Design review of the part built by this model. Coordinates are the model's own, in mm. A direction names the side the tool comes from. Round coordinates to 2 decimals unless told otherwise and drop trailing zeros. Loops run counter-clockwise (first coordinate to the right, second up) from the corner with the lowest first, then second, coordinate; pieces in that order, holes last. Notation, with made-up numbers: (-32, 84.25) - (-27, 84.25) arc R7 cw to (-27, 90.25) - close; hole circle Ø6 at (75.5, 44). An arc over 180 degrees is marked (long way). Return JSON: item names as keys, results as strings. Group by question number.
(1) We need section B-B, the plane y = 13.2. Write out the cut boundary in (x, z).
(2) For faces 5 (the flat face through (27, 25, 1.5)), 6 (the cylindrical face through (-0.2, 13.1, 9.6)), 7 (the flat face through (1, 3, 2.2)), 8 (the flat face through (21, 22.4, -1)), list the 3-axis set-ups (+Z, -Z, +X, -X, +Y, -Y) from which the entire face can be reached by the end or side of a thin tool; tool diameter is ignored.
(3) We need section A-A, the plane x = 14. Write out the cut boundary in (y, z).
(4) The part is to be moulded in two halves that separate along X. For faces 1 (the flat face through (1.3, 12, 7)), 2 (the flat face through (22, 2, -1)), 3 (the flat face through (-0.7, 12, 0)), 4 (the flat face through (21, 25, -1.5)), say which applies: pulls with the +X half, pulls with the -X half, needs draft (parallel to the pull), parting line crosses it, or undercut.
(5) We need section C-C, the plane x = 40.5. Write out the cut boundary in (y, z), and give its area (3 significant figures).
(6) Wall thickness on L1, parallel to Y at x = 16.5, z = 1.25; L2, parallel to X at y = 9.75, z = -1; L3, parallel to X at y = 1, z = 5: over which ranges is each line inside the solid? List them lowest first. Write a range as [from, to].
(7) Clearance check with flat-ended pins moving along their axes: pin 1 (6 mm diameter, centred on x = 38, y = 8, fed in from +Z); pin 2 (6.5 mm diameter, centred on y = 11.5, z = 5.5, fed in from -X). State where each tip first meets the part, or that it passes through.
(8) We need section D-D, the plane z = 9. Write out the cut boundary in (x, y), and give its area (3 significant figures).
Autodesk Fusion 360 part; units mm, degrees
sketch "Sketch1" plane through (0, 0, 0) normal (0, 0, 1) x (1, 0, 0)
  line L0 (0, 0) -> (42, 0)
  line L1 (42, 0) -> (42, 24.4)
  line L2 (42, 24.4) -> (0, 24.4)
  line L3 (0, 24.4) -> (0, 0)
  line L4 (-0.2, 24.6) -> (42.2, 24.6)
  line L5 (42.2, 24.6) -> (42.2, -0.2)
  line L6 (42.2, -0.2) -> (-0.2, -0.2)
  line L7 (-0.2, -0.2) -> (-0.2, 24.6)
  line L8 (-0.7, 26.1) -> (43.7, 26.1)
  line L9 (43.7, 26.1) -> (43.7, -1.7)
  line L10 (43.7, -1.7) -> (-0.7, -1.7)
  line L11 (-0.7, -1.7) -> (-0.7, 26.1)
  line L12 (-0.7, 26.1) -> (1.3, 26.1)
  line L13 (1.3, 26.1) -> (1.3, -1.7)
  line L14 (1.3, -1.7) -> (-0.7, -1.7)
  line L15 (-0.7, -1.7) -> (-0.7, 26.1)
  line L16 (3.3, 22.4) -> (40, 22.4)
  line L17 (40, 22.4) -> (40, 2)
  line L18 (40, 2) -> (3.3, 2)
  line L19 (3.3, 2) -> (3.3, 22.4)
  dimension "d1" = 42
  dimension "d2" = 24.4
  dimension "d3" = 0.2
  dimension "d4" = 0.2
  dimension "d5" = 0.2
  dimension "d6" = 0.2
  dimension "d7" = 0.5
  dimension "d8" = 1.5
  dimension "d9" = 1.5
  dimension "d10" = 1.5
  dimension "d11" = 2
  dimension "d12" = 27.8
  dimension "d13" = 2
  dimension "d14" = 2
  dimension "d15" = 2
  dimension "d16" = 2
extrude "Extrude1" add sketch "Sketch1" against normal blind 1.5
extrude "Extrude2" add sketch "Sketch1" along normal blind 1.5 contours L4 L5 L6 L8 L9 L10 L13
extrude "Extrude3" add sketch "Sketch1" along normal blind 10 contours L4 L6 L7 L8 L10 L11 L12 L13 L14 L15
sketch "Sketch2" plane through (-0.7, 0, 0) normal (-1, 0, 0) x (0, -1, 0)
  line L0 (-26.1, 10) -> (-26.1, -1.5)
  line L1 (-26.1, -1.5) -> (1.7, -1.5)
  line L2 (1.7, -1.5) -> (1.7, 10)
  line L3 (1.7, 10) -> (-26.1, 10)
  line L4 (-24.4, 0) -> (0, 0)
  line L5 (0, 0) -> (0, 1.2)
  line L6 (0, 1.2) -> (-24.4, 1.2)
  line L7 (-24.4, 1.2) -> (-24.4, 0)
  line L8 (-19.6, 1.2) -> (-4.8, 1.2)
  line L9 (-4.8, 1.2) -> (-4.8, 3.2)
  line L10 (-4.8, 3.2) -> (-19.6, 3.2)
  line L11 (-19.6, 3.2) -> (-19.6, 1.2)
  line L12 (-4.8, 3.2) -> (-6.8, 3.2)
  line L13 (-6.8, 3.2) -> (-6.8, 1.2)
  line L14 (-6.8, 1.2) -> (-4.8, 1.2)
  line L15 (-4.8, 1.2) -> (-4.8, 3.2)
  circle A0 centre (-13.2, 3.2) radius 6.4
  dimension "d23" = 24.4
  dimension "d24" = 1.2
  dimension "d25" = 1.7
  dimension "d26" = 14.8
  dimension "d27" = 2
  dimension "d28" = 4.8
  dimension "d29" = 2
  dimension "d30" = 2
  dimension "d31" = 12.8
  dimension "d32" = 6.4
extrude "Extrude4" add sketch "Sketch2" against normal blind 2 contours L0 L1 L2 L3 L4 L5 L6 L7 L9 L10 L11 L12 L15 A0 | L1 L4 A0 | L10 A0 | L6 L8 L9 L10 L12 L13 L14 L15
extrude "Extrude5" cut sketch "Sketch2" against normal blind 1 contours L6 L8 L10 A0 | L6 L8 L11 A0 | L6 L8 L13 A0 | L10 A0
extrude "Extrude6" cut 1 faces at (0.3, 24.4, 0.8) along direction (0, 1, 0) blind 0.2
extrude "Extrude7" cut 1 faces at (0.3, 0, 0.4) along direction (0, -1, 0) blind 0.2
extrude "Extrude8" cut 2 faces at (0.8, 4.4667, 1.2) (0.8, 22.9333, 1.2) along direction (0, 0, 1) blind 0.5
extrude "Extrude9" cut 1 faces at (0.9667, 11.0667, 3.2) along direction (0, 0, 1) blind 0.5
extrude "Extrude10" cut 2 faces at (0.8, 4.4667, 1.7) (0.8, 22.9333, 1.7) along direction (0, 0, 1) blind 0.5
equation "d25 = ( 3.4 / 2 ) * 1 mm"
equation "d28 = ( 9.6 / 2 ) * 1 mm"
Solutions:
{
 "1": {"outline": "(-0.7, -1.5) - (3.3, -1.5) - (3.3, 0) - (-0.2, 0) - (-0.2, 1.2) - (-0.7, 1.2) - close; (-0.7, 9.6) - (0.3, 9.6) - (0.3, 3.7) - (1.3, 3.7) - (1.3, 10) - (-0.7, 10) - close; (40, -1.5) - (43.7, -1.5) - (43.7, 1.5) - (42.2, 1.5) - (42.2, 0) - (40, 0) - close"},
 "2": {"face 5": "+Z, +X, +Y, -Y", "face 6": "-X", "face 7": "+X", "face 8": "+Z, -Z"},
 "3": {"outline": "(-1.7, -1.5) - (2, -1.5) - (2, 0) - (-0.2, 0) - (-0.2, 1.5) - (-1.7, 1.5) - close; (22.4, -1.5) - (26.1, -1.5) - (26.1, 1.5) - (24.6, 1.5) - (24.6, 0) - (22.4, 0) - close"},
 "4": {"face 1": "pulls with the +X half", "face 2": "undercut", "face 3": "pulls with the -X half", "face 4": "needs draft"},
 "5": {"outline": "(-1.7, -1.5) - (26.1, -1.5) - (26.1, 1.5) - (24.6, 1.5) - (24.6, 0) - (-0.2, 0) - (-0.2, 1.5) - (-1.7, 1.5) - close", "area": "46.2 mm^2"},
 "6": {"L1": "[-1.7, -0.2], [24.6, 26.1]", "L2": "[-0.7, 3.3], [40, 43.7]", "L3": "[-0.7, 1.3]"},
 "7": {"pin 1": "z = 0", "pin 2": "x = 0.3"},
 "8": {"outline": "(-0.7, -1.7) - (1.3, -1.7) - (1.3, 26.1) - (-0.7, 26.1) - (-0.7, 15.91) - (0.3, 15.91) - (0.3, 10.49) - (-0.7, 10.49) - close", "area": "50.2 mm^2"}
}
